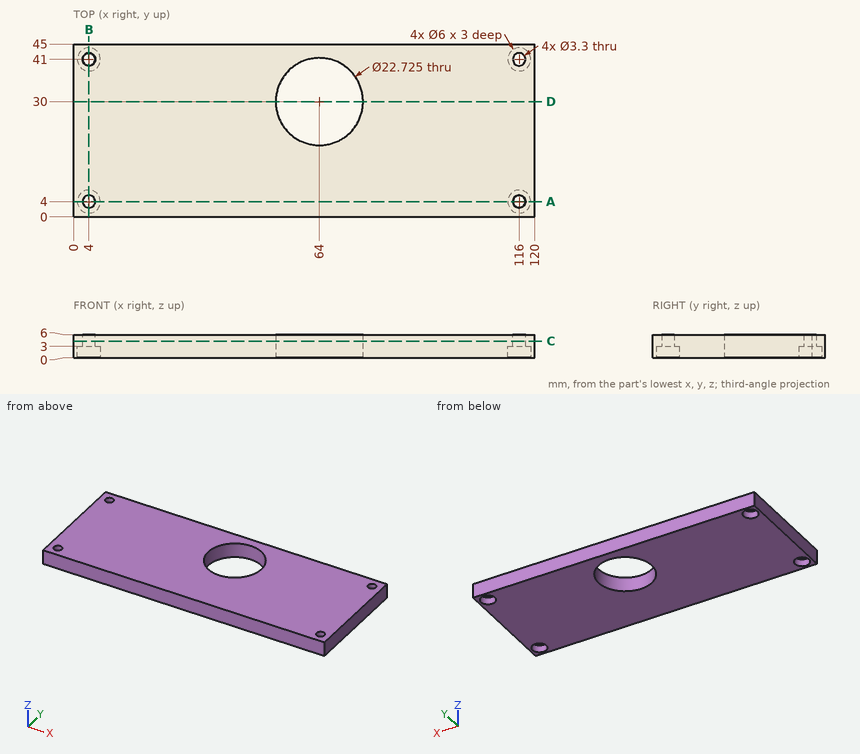
Check sheet for the drawn part. Datum: minimum x, y, z corner. Units: mm. Round coordinates to 2 decimals unless told otherwise and drop trailing zeros. Order: outer loops, then holes, each group sorted by start corner. A loop starts at its lowest first (then second) coordinate and runs counter-clockwise, first axis right, second up. Notation, with made-up numbers: (-0.5, 65.5) -> (22.5, 65.5) arc R12 ccw to (22.5, 82.5) -> close; hole circle Ø7 at (38.5, 50). An arc over 180 degrees is marked (long way). Put each result on its own line as item: value. Start each with the question number.
(1) Section check A-A (y = 4). Enter the section's corners in (x, z), then the cut area to 3 significant figures.
(2) Material ranges on line 1 along Y through (x, z) = (4, 5.05); line 2 along X through (y, z) = (4, 2.15); line 3 along X through (y, z) = (42.5, 5.55), recorded low to high.
(3) Section check D-D (y = 30). Enter the section's corners in (x, z).
(4) Section check C-C (z = 4.4). State how many separate pieces and enclosed holes the cut face has, then the cut area to 3 significant figures.
(5) Depth check by flat-ended pin: pin 1 Ø2.5 at (x, y) = (4, 4) entering from +Z; pin 2 Ø8 at (x, y) = (53.5, 13) entering from -Z; pin 3 Ø3.5 at (x, y) = (116, 4) entering from -Z. Enter the tip coordinate at first touch or a pass-through.
(6) Section check B-B (x = 4). Enter the section's corners in (y, z).
Completed:
1. outline: (0, 0) -> (1, 0) -> (1, 3) -> (2.35, 3) -> (2.35, 6) -> (0, 6) -> close; (5.65, 3) -> (7, 3) -> (7, 0) -> (113, 0) -> (113, 3) -> (114.35, 3) -> (114.35, 6) -> (5.65, 6) -> close; (117.65, 3) -> (119, 3) -> (119, 0) -> (120, 0) -> (120, 6) -> (117.65, 6) -> close
1. area: 664 mm2
2. line 1: y = 0 to 2.35, 5.65 to 39.35, 42.65 to 45
2. line 2: x = 0 to 1, 7 to 113, 119 to 120
2. line 3: x = 0 to 3.31, 4.69 to 115.31, 116.69 to 120
3. outline: (0, 0) -> (52.64, 0) -> (52.64, 6) -> (0, 6) -> close; (75.36, 0) -> (120, 0) -> (120, 6) -> (75.36, 6) -> close
4. separate pieces: 1
4. enclosed holes: 5
4. area: 4,960 mm2
5. pin 1: passes through
5. pin 2: stops at z = 0
5. pin 3: stops at z = 3
6. outline: (0, 0) -> (1, 0) -> (1, 3) -> (2.35, 3) -> (2.35, 6) -> (0, 6) -> close; (5.65, 3) -> (7, 3) -> (7, 0) -> (38, 0) -> (38, 3) -> (39.35, 3) -> (39.35, 6) -> (5.65, 6) -> close; (42.65, 3) -> (44, 3) -> (44, 0) -> (45, 0) -> (45, 6) -> (42.65, 6) -> close
